```python
from build123d import *

# Parameters (mm, degrees)
BOSS_EXTRUDE1_DEPTH      = 8
BOSS_EXTRUDE1_DEPTH_BACK = 8
SKETCH2_R                = 2
CUT_EXTRUDE1_DEPTH       = 2
CUT_EXTRUDE2_START       = -2
CUT_EXTRUDE2_DEPTH       = 2
BOSS_EXTRUDE4_DEPTH      = 16
CUT_EXTRUDE4_DEPTH       = 2
CUT_EXTRUDE4_DEPTH_BACK  = 2
BOSS_EXTRUDE6_DEPTH      = 13
BOSS_EXTRUDE6_DEPTH_BACK = 13
SKETCH12_W               = 46
SKETCH12_H               = 5.136814738
SKETCH13_R               = 1.25
CUT_EXTRUDE5_DEPTH       = 16
BOSS_EXTRUDE7_DEPTH      = 26
SKETCH15_W               = 3
SKETCH15_H               = 26
BOSS_EXTRUDE8_DEPTH      = 3
SKETCH20_W               = 2.5
SKETCH20_H               = 4
CUT_EXTRUDE8_DEPTH       = 57.520887153
BOSS_EXTRUDE9_DEPTH      = 5.14
CUT_EXTRUDE9_START       = -5.14
CUT_EXTRUDE9_DEPTH       = 5.14
BOSS_EXTRUDE10_DEPTH     = 5.14
CUT_EXTRUDE10_DEPTH      = 5.14
SKETCH25_W               = 26.5
SKETCH25_H               = 22.5
CUT_EXTRUDE11_DEPTH      = 2.25
SKETCH26_W               = 3
SKETCH26_H               = 5
CUT_EXTRUDE12_DEPTH      = 3


with BuildPart() as part:
    # Sketch2 → Boss-Extrude1 (new, two sides: drawn at the far end of the back side and taken through both)
    with BuildSketch(Plane(origin=(0, 0, 0), x_dir=(1, 0, 0), z_dir=(0, 1, 0)).offset(-BOSS_EXTRUDE1_DEPTH_BACK)):
        with BuildLine():
            Line((-8.523572923, 1.405956139), (-14.862846849, -12.188660667))
            ThreePointArc((-14.862846849, -12.188660667), (-15.958655574, -13.708165939), (-17.536798633, -14.717699254))
            Line((-17.536798633, -14.717699254), (-19.186952062, -14.717699254))
            Line((-19.186952062, -14.717699254), (-21.263787389, -14.712954143))
            Line((-21.263787389, -14.712954143), (-31.98936925, -14.712954143))
            ThreePointArc((-31.98936925, -14.712954143), (-25.026485616, -6.579447275), (-31.98936925, 1.554059594))
            Line((-31.98936925, 1.554059594), (-31.98936925, 2.123860595))
            Line((-31.98936925, 2.123860595), (-25.889500724, 3.009865365))
            Line((-25.889500724, 3.009865365), (-15.1825186, 8.043883417))
            ThreePointArc((-15.1825186, 8.043883417), (-9.525170989, 7.060165556), (-8.523572923, 1.405956139))
        make_face()
        with Locations(Location((-19.394385785, -10.075569358, 0), (0, 0, 270))):
            Circle(SKETCH2_R, mode=Mode.SUBTRACT)
        with Locations(Location((-13.055111858, 3.519047448, 0), (0, 0, 270))):
            Circle(SKETCH2_R, mode=Mode.SUBTRACT)
    extrude(amount=BOSS_EXTRUDE1_DEPTH + BOSS_EXTRUDE1_DEPTH_BACK)

    # Sketch3 → Cut-Extrude1 (cut)
    with BuildSketch(Plane.XZ.offset(8)):
        with BuildLine():
            Line((-13.383682933, 9.016583412), (-36.019194906, -1.538529167))
            Line((-36.019194906, -1.538529167), (-25.889500724, -3.009865365))
            Line((-25.889500724, -3.009865365), (-15.1825186, -8.043883417))
            ThreePointArc((-15.1825186, -8.043883417), (-9.525170989, -7.060165556), (-8.523572923, -1.405956139))
            Line((-8.523572923, -1.405956139), (-13.383682933, 9.016583412))
        make_face()
    extrude(amount=-CUT_EXTRUDE1_DEPTH, mode=Mode.SUBTRACT)

    # Sketch4 → Cut-Extrude2 (cut)
    with BuildSketch(Plane(origin=(0, 8, 0), x_dir=(1, 0, 0), z_dir=(0, 1, 0)).offset(CUT_EXTRUDE2_START)):
        with BuildLine():
            Line((-13.383682933, -9.016583412), (-36.019194906, 1.538529167))
            Line((-36.019194906, 1.538529167), (-25.889500724, 3.009865365))
            Line((-25.889500724, 3.009865365), (-15.1825186, 8.043883417))
            ThreePointArc((-15.1825186, 8.043883417), (-9.525170989, 7.060165556), (-8.523572923, 1.405956139))
            Line((-8.523572923, 1.405956139), (-13.383682933, -9.016583412))
        make_face()
    extrude(amount=CUT_EXTRUDE2_DEPTH, mode=Mode.SUBTRACT)

    # Sketch7 → Boss-Extrude4 (add)
    with BuildSketch(Plane.XZ.offset(8)):
        with BuildLine():
            Line((-31.98936925, -1.554059594), (-31.98936925, 14.712954143))
            ThreePointArc((-31.98936925, 14.712954143), (-26.036622944, 10.530440134), (-25.724576966, 3.261930016))
            ThreePointArc((-25.724576966, 3.261930016), (-28.241329009, 0.053085809), (-31.98936925, -1.554059594))
        make_face()
    extrude(amount=-BOSS_EXTRUDE4_DEPTH)

    # Sketch10 → Cut-Extrude4 (cut, two sides: drawn at the far end of the back side and taken through both)
    with BuildSketch(Plane(origin=(0, 0, 0), x_dir=(1, 0, 0), z_dir=(0, 1, 0)).offset(-CUT_EXTRUDE4_DEPTH_BACK)):
        with BuildLine():
            Line((-25.889500724, 3.009865365), (-15.1825186, 8.043883417))
            ThreePointArc((-15.1825186, 8.043883417), (-9.525170989, 7.060165556), (-8.523572923, 1.405956139))
            Line((-8.523572923, 1.405956139), (-13.383682933, -9.016583412))
            Line((-13.383682933, -9.016583412), (-25.724576966, -3.261930016))
            ThreePointArc((-25.724576966, -3.261930016), (-28.241329009, -0.053085809), (-31.98936925, 1.554059594))
            Line((-31.98936925, 1.554059594), (-31.98936925, 2.123860595))
            Line((-31.98936925, 2.123860595), (-25.889500724, 3.009865365))
        make_face()
    extrude(amount=CUT_EXTRUDE4_DEPTH + CUT_EXTRUDE4_DEPTH_BACK, mode=Mode.SUBTRACT)

    # Sketch12 → Boss-Extrude6 (add, two sides: drawn at the far end of the back side and taken through both)
    with BuildSketch(Plane(origin=(0, 0, 0), x_dir=(1, 0, 0), z_dir=(0, 1, 0)).offset(-BOSS_EXTRUDE6_DEPTH_BACK)):
        with Locations((-54.98936925, -0.444546774)):
            Rectangle(SKETCH12_W, SKETCH12_H)
    extrude(amount=BOSS_EXTRUDE6_DEPTH + BOSS_EXTRUDE6_DEPTH_BACK)

    # Sketch13 → Cut-Extrude5 (cut)
    with BuildSketch(Plane.XZ.offset(8)):
        with Locations(Location((-28.48936925, 11.462954143, 0), (0, 0, 270))):
            Circle(SKETCH13_R)
    extrude(amount=-CUT_EXTRUDE5_DEPTH, mode=Mode.SUBTRACT)

    # Sketch14 → Boss-Extrude7 (add)
    with BuildSketch(Plane.XZ.offset(13)):
        with BuildLine():
            Line((-81.98936925, 8.012954143), (-84.98936925, 8.012954143))
            add(Edge.make_bspline(
                [(-77.98936925, -2.123860595), (-83.929409171, 2.617289227), (-84.98936925, 8.012954143)],
                knots=[0, 0, 0, 0.697154263, 0.697154263, 0.697154263], degree=2))
            Line((-77.98936925, -2.123860595), (-77.98936925, 3.012954143))
            add(Edge.make_bspline(
                [(-77.98936925, 3.012954143), (-81.112416602, 5.119010403), (-81.98936925, 8.012954143)],
                knots=[0, 0, 0, 0.561523676, 0.561523676, 0.561523676], degree=2))
        make_face()
    extrude(amount=-BOSS_EXTRUDE7_DEPTH)

    # Sketch15 → Boss-Extrude8 (add)
    with BuildSketch(Plane.XY.offset(3.012954143)):
        with Locations((-40.23936925, 0)):
            Rectangle(SKETCH15_W, SKETCH15_H)
        with Locations((-69.73936925, 0)):
            Rectangle(SKETCH15_W, SKETCH15_H)
    extrude(amount=BOSS_EXTRUDE8_DEPTH)

    # Sketch20 → Cut-Extrude8 (cut, through all)
    with BuildSketch(Plane.ZY.offset(31.98936925)):
        with Locations((3.021305608, 0)):
            Rectangle(SKETCH20_W, SKETCH20_H)
    extrude(amount=-CUT_EXTRUDE8_DEPTH, mode=Mode.SUBTRACT)

    # Sketch21 → Boss-Extrude9 (add)
    with BuildSketch(Plane(origin=(0, 0, -2.123860595), x_dir=(-1, 0, 0), z_dir=(0, 0, -1))):
        with BuildLine():
            Line((26.98936925, 8), (31.98936925, 8))
            Line((31.98936925, 8), (31.98936925, 13))
            ThreePointArc((31.98936925, 13), (28.453835344, 11.535533906), (26.98936925, 8))
        make_face()
    extrude(amount=-BOSS_EXTRUDE9_DEPTH)

    # Sketch22 → Cut-Extrude9 (cut)
    with BuildSketch(Plane(origin=(0, 13, 0), x_dir=(1, 0, 0), z_dir=(0, 1, 0)).offset(CUT_EXTRUDE9_START)):
        with BuildLine():
            Line((-31.98936925, 2.123860595), (-31.98936925, 1.554059594))
            ThreePointArc((-31.98936925, 1.554059594), (-29.238037233, 0.603941382), (-26.98936925, -1.244313143))
            Line((-26.98936925, -1.244313143), (-26.98936925, 2.123860595))
            Line((-26.98936925, 2.123860595), (-31.98936925, 2.123860595))
        make_face()
    extrude(amount=CUT_EXTRUDE9_DEPTH, mode=Mode.SUBTRACT)

    # Sketch23 → Boss-Extrude10 (add)
    with BuildSketch(Plane(origin=(0, 0, -2.123860595), x_dir=(-1, 0, 0), z_dir=(0, 0, -1))):
        with BuildLine():
            Line((31.98936925, -8), (31.98936925, -13))
            ThreePointArc((31.98936925, -13), (28.453835344, -11.535533906), (26.98936925, -8))
            Line((26.98936925, -8), (31.98936925, -8))
        make_face()
    extrude(amount=-BOSS_EXTRUDE10_DEPTH)

    # Sketch24 → Cut-Extrude10 (cut)
    with BuildSketch(Plane.XZ.offset(13)):
        with BuildLine():
            Line((-31.98936925, -1.554059594), (-31.98936925, -2.123860595))
            Line((-31.98936925, -2.123860595), (-25.837669131, -2.123860595))
            Line((-25.837669131, -2.123860595), (-25.837669131, 3.016139405))
            ThreePointArc((-25.837669131, 3.016139405), (-26.35642668, 2.093115722), (-26.98936925, 1.244313143))
            ThreePointArc((-26.98936925, 1.244313143), (-29.238037233, -0.603941382), (-31.98936925, -1.554059594))
        make_face()
    extrude(amount=-CUT_EXTRUDE10_DEPTH, mode=Mode.SUBTRACT)

    # Sketch25 → Cut-Extrude11 (cut)
    with BuildSketch(Plane.XY.offset(3.012954143)):
        with Locations((-54.98936925, 0)):
            Rectangle(SKETCH25_W, SKETCH25_H)
    extrude(amount=-CUT_EXTRUDE11_DEPTH, mode=Mode.SUBTRACT)

    # Sketch26 → Cut-Extrude12 (cut)
    with BuildSketch(Plane.XY.offset(6.012954143)):
        with Locations((-40.23936925, 0)):
            Rectangle(SKETCH26_W, SKETCH26_H)
    extrude(amount=-CUT_EXTRUDE12_DEPTH, mode=Mode.SUBTRACT)


solid = part.part
```
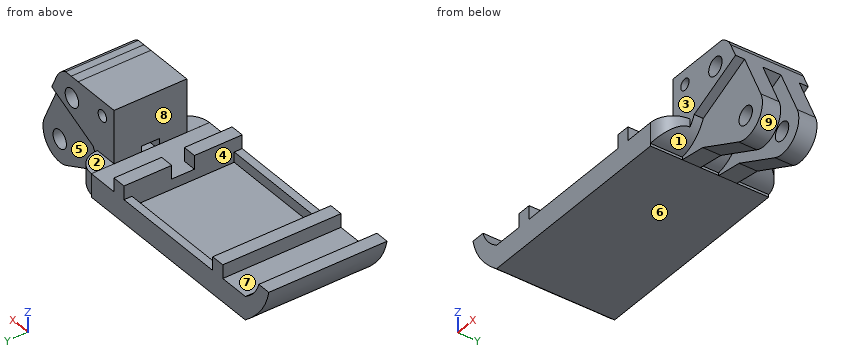
Check sheet for the modelled part. Datum: model origin and axes. Units: mm. Face numbers are marked on the shaded views. A direction names the side the tool comes from. Round coordinates to 2 decimals unless told otherwise and drop trailing zeros. Loops run counter-clockwise (first coordinate to the right, second up) from the corner with the lowest first, then second, coordinate; pieces in that order, holes last. Notation, with made-up numbers: M 46,81 L 99,81 A16 ccw 99,98 Z; hole C 6,87.5 d7. An arc over 180 degrees is marked long. Answer as a JSON object with one key per item and string values.
1. Gauge pin test, flat ends, axial feed: P1, Ø3.5, axis at x = -40, y = -6, coming from the +Z side; P2, Ø2.5, axis at x = -29.5, y = -10, coming from the +Z side; P3, Ø1, axis at x = -52, y = -6, coming from the +Z side; P4, Ø12, axis at x = -25, y = 0.5, coming from the +Z side. Record the tip position at first contact, or that the pin passes through.
Reply:
{"P1": "stops at z = 6.01", "P2": "stops at z = 3.02", "P3": "stops at z = 0.76", "P4": "stops at z = 14.72"}
2. Section check D-D (x = -24.5). Record the boundary of the cut face in (y, z), plus the area to 3 significant figures.
Reply:
{"outline": "M -8,3.83 L -6,3.83 L -6,-3.66 L -2,-3.66 L -2,4.27 L 2,4.27 L 2,-3.66 L 6,-3.66 L 6,3.83 L 8,3.83 L 8,14.71 L -8,14.71 Z", "area": "232 mm²"}
3. Access from +Z, -Z, +X, -X, +Y, -Y to the whole of each face (thin tool, end or side, straight path). Record for the marked faces 1, 2, 3, 4 and 5.
Reply:
{"face 1": "-Z, +X, -Y", "face 2": "+Z, +X, +Y", "face 3": "+Z, +X, -Y", "face 4": "+Z", "face 5": "-Z, +X, +Y"}
4. Section check C-C (y = 3.75). State how many separate pieces and enclosed holes the cut face has, plus the area to 3 significant figures.
Reply:
{"separate pieces": "1", "enclosed holes": "3", "area": "609 mm²"}
5. Section check B-B (z = 11.25). Record the boundary of the cut face in (x, y).
Reply:
{"outline": "M -31.99,-8 L -29.72,-8 L -29.72,8 L -31.99,8 Z; M -27.26,-8 L -21.01,-8 L -21.01,8 L -27.26,8 Z; M -17.78,-8 L -14.43,-8 L -14.43,8 L -17.78,8 Z"}
6. Section check A-A (x = -67.5). Record the boundary of the cut face in (y, z).
Reply:
{"outline": "M -13,-2.12 L 13,-2.12 L 13,3.01 L 11.25,3.01 L 11.25,0.76 L -11.25,0.76 L -11.25,3.01 L -13,3.01 Z"}
7. Mould release check, pull along X, two halves, no side actions. Record for the marked faces 6, 7, 8 and 9: pulls with the +X half, pulls with the -X half, needs draft (parallel to the pull), parting line crosses it, or undercut.
Reply:
{"face 6": "needs draft", "face 7": "undercut", "face 8": "undercut", "face 9": "parting line crosses it"}
8. Scan lines: line 1 (X direction, y = -5.5, z = 3.25); line 2 (X direction, y = 4.5, z = 11); line 3 (Z direction, x = -76, y = -0.5). Record each from-to range of solid material in increasing order.
Reply:
{"line 1": "x = -83.02 to -78.33, -71.24 to -68.24, -41.74 to -38.74, -31.99 to -10.69", "line 2": "x = -31.99 to -29.65, -27.33 to -21.17, -17.62 to -14.31", "line 3": "z = -2.12 to 3.01"}
